The model under review builds one solid part; all positions refer to its coordinate system, in mm. A direction names the side the tool comes from. Round coordinates to 2 decimals unless told otherwise and drop trailing zeros. Use CSV: the item, a comma, the result in double quotes. Start each with the question number.
1) Machinability: for faces 4 (the face through (42, -26.5, 9)), 5 (the face through (42, 593.5, 9)), 6 (the face through (183, 603.5, 9)), which of the approach directions +Z, -Z, +X, -X, +Y, -Y give a long, thin tool a straight path to every point of the face, cutting with its end or side? Answer none if there is none.
2) Wall thickness on probe 1 along Y at (x, z) = (2.2, 6.25); probe 2 along Y at (x, z) = (10.85, 10); probe 3 along X at (y, z) = (190.5, 11.25): over which ranges is each line inside the solid? List them lowest first. Write a range as [from, to].
3) Mouldability with a two-part tool opening along X and no side actions: class faces 1 (the face through (11, 603.5, 9)), 2 (the face through (-5.3, 279, 9)), 3 (the face through (152, -26.5, 9)) as released by +X, released by -X, zero draft, split by the parting line, or undercut.
from build123d import *

# Parameters (mm, degrees)
SKETCH1_W                = 204.6
SKETCH1_H                = 640
BOSS_EXTRUDE1_DEPTH      = 18
SKETCH4_W                = 30
SKETCH4_H                = 10
CUT_EXTRUDE1_DEPTH       = 18
F_3_0_3_DIAMETER_HOLE3_D = 3
F_3_0_3_DIAMETER_HOLE5_D = 3


with BuildPart() as part:
    # Sketch1 → Boss-Extrude1 (new body)
    with BuildSketch(Plane.XY):
        with Locations((97, 283.5)):
            Rectangle(SKETCH1_W, SKETCH1_H)
    extrude(amount=BOSS_EXTRUDE1_DEPTH)

    # Sketch4 → Cut-Extrude1 (cut)
    with BuildSketch(Plane(origin=(0, 0, 0), x_dir=(-1, 0, 0), z_dir=(0, 0, -1))):
        with Locations((-42, -31.5)):
            Rectangle(SKETCH4_W, SKETCH4_H)
        with Locations((-152, -31.5)):
            Rectangle(SKETCH4_W, SKETCH4_H)
        with Locations((-42, 598.5)):
            Rectangle(SKETCH4_W, SKETCH4_H)
        with Locations((-152, 598.5)):
            Rectangle(SKETCH4_W, SKETCH4_H)
    extrude(amount=-CUT_EXTRUDE1_DEPTH, mode=Mode.SUBTRACT)

    # Ø3.0 (3) Diameter Hole3 (through all)
    with Locations(Plane(origin=(0, 0, 0), x_dir=(-1, 0, 0), z_dir=(0, 0, -1))):
        with Locations((-2.2, 190.5), (-2.2, -1.5), (-191.8, -1.5), (-191.8, 190.5), (-191.8, 478.5), (-2.2, 478.5)):
            Hole(F_3_0_3_DIAMETER_HOLE3_D / 2)

    # Ø3.0 (3) Diameter Hole5 (through all)
    with Locations(Plane(origin=(0, 0, 0), x_dir=(-1, 0, 0), z_dir=(0, 0, -1))):
        with Locations((238.536571684, 43.354956744), (-97, -31.5), (-183.15, -31.5), (-10.85, -31.5), (-10.85, 598.5), (-183.15, 598.5), (-97, 598.5)):
            Hole(F_3_0_3_DIAMETER_HOLE5_D / 2)


solid = part.part
Values found:
1,face 4,"+Z, -Z, -Y"
1,face 5,"+Z, -Z, +Y"
1,face 6,"+Z, -Z, +X, -X, +Y"
2,probe 1,"[-36.5, -3], [0, 189], [192, 477], [480, 603.5]"
2,probe 2,"[-36.5, -33], [-30, 597], [600, 603.5]"
2,probe 3,"[-5.3, 0.7], [3.7, 190.3], [193.3, 199.3]"
3,face 1,"zero draft"
3,face 2,"released by -X"
3,face 3,"undercut"
